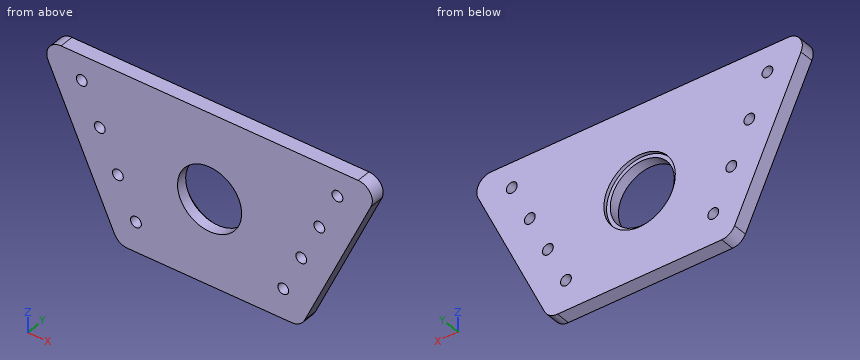
```python
from build123d import *

# Parameters (mm, degrees)
SKETCH1_R           = 14.2875
BOSS_EXTRUDE1_DEPTH = 6.35
SKETCH2_R           = 2.413
CUT_EXTRUDE1_DEPTH  = 86.430512699
FILLET1_R           = 6.35
SKETCH3_R           = 15.9385
CUT_EXTRUDE2_DEPTH  = 1.5875


with BuildPart() as part:
    # Sketch1 → Boss-Extrude1 (new body)
    with BuildSketch(Plane(origin=(0, 0, 0), x_dir=(1, 0, 0), z_dir=(0, 1, 0))):
        Polygon((-40.667356449, 38.1), (40.667356449, 38.1), (76.2, -38.1), (-76.2, -38.1), align=None)
        with Locations(Location((0, 0, 0), (0, 0, 270))):
            Circle(SKETCH1_R, mode=Mode.SUBTRACT)
    extrude(amount=BOSS_EXTRUDE1_DEPTH)

    # Sketch2 → Cut-Extrude1 (cut, through all)
    with BuildSketch(Plane(origin=(0, 6.35, 0), x_dir=(1, 0, 0), z_dir=(0, 1, 0))):
        with Locations(Location((-57.005256578, -26.9875, 0), (0, 0, 270))):
            Circle(SKETCH2_R)
        with Locations(Location((-48.954378692, -9.722336657, 0), (0, 0, 270))):
            Circle(SKETCH2_R)
        with Locations(Location((-40.903500806, 7.542826686, 0), (0, 0, 270))):
            Circle(SKETCH2_R)
        with Locations(Location((-32.852622919, 24.807990029, 0), (0, 0, 270))):
            Circle(SKETCH2_R)
        with Locations(Location((32.852622919, 24.807990029, 0), (0, 0, 90))):
            Circle(SKETCH2_R)
        with Locations(Location((40.903500806, 7.542826686, 0), (0, 0, 90))):
            Circle(SKETCH2_R)
        with Locations(Location((48.954378692, -9.722336657, 0), (0, 0, 90))):
            Circle(SKETCH2_R)
        with Locations(Location((57.005256578, -26.9875, 0), (0, 0, 90))):
            Circle(SKETCH2_R)
    extrude(amount=-CUT_EXTRUDE1_DEPTH, mode=Mode.SUBTRACT)

    # Fillet1
    fillet1_edges = [part.edges().sort_by_distance(p)[0] for p in [
        (-40.667356449, 3.175, -38.1),
        (40.667356449, 3.175, -38.1),
        (76.2, 3.175, 38.1),
        (-76.2, 3.175, 38.1),
    ]]
    fillet(fillet1_edges, radius=FILLET1_R)

    # Sketch3 → Cut-Extrude2 (cut)
    with BuildSketch(Plane(origin=(0, 6.35, 0), x_dir=(1, 0, 0), z_dir=(0, 1, 0))):
        with Locations(Location((0, 0, 0), (0, 0, 270))):
            Circle(SKETCH3_R)
    extrude(amount=-CUT_EXTRUDE2_DEPTH, mode=Mode.SUBTRACT)


solid = part.part
```
Input: part model. Units: mm. Frame: model coordinates. Give positions to 0.01 mm unless a question says otherwise; leave off trailing zeros. Order: outer loops, then holes, each group sorted by start corner. A loop starts at its lowest first (then second) coordinate and runs counter-clockwise, first axis right, second up. Notation, with made-up numbers: (10.25, -38) - (47.25, -38) arc R31 ccw to (47.25, -11) - close; hole circle Ø6 at (87.5, -7). An arc over 180 degrees is marked (long way). Use a Markdown table: item, result.
(1) Section query A-A (x = 0). Output: boundary loops of the cut face in (y, z).
Computed values:
| item | result |
|---|---|
| outline | (0, -38.1) - (6.35, -38.1) - (6.35, -15.94) - (4.76, -15.94) - (4.76, -14.29) - (0, -14.29) - close; (0, 14.29) - (4.76, 14.29) - (4.76, 15.94) - (6.35, 15.94) - (6.35, 38.1) - (0, 38.1) - close |
(2) Section query C-C (y = 2.25). State how many separate pieces and enclosed holes the cut face has, then the cut area to 3 significant figures.
Computed values:
| item | result |
|---|---|
| separate pieces | 1 |
| enclosed holes | 9 |
| area | 8,070 mm2 |
(3) Pin query (flat end, axial travel): pin 1 (23 mm diameter, centred on x = 0, z = 0, fed in from +Y); pin 2 (2 mm diameter, centred on y = 2, z = 27.5, fed in from -X). Return the tip coordinate at first contact, or that it passes through.
Computed values:
| item | result |
|---|---|
| pin 1 | passes through |
| pin 2 | stops at x = -71.72 |
(4) Line query: line 1 (X direction, y = 3, z = -9); line 2 (X direction, y = 0.75, z = -27); line 3 (X direction, y = 2.5, z = 25). Output: solid intervals per line, ascending. Write a range as from..to.
Computed values:
| item | result |
|---|---|
| line 1 | x = -54.24..-42.83, -38.98..-11.1, 11.1..38.98, 42.83..54.24 |
| line 2 | x = -45.84..-33.86, -31.84..31.84, 33.86..45.84 |
| line 3 | x = -70.09..-58.37, -55.64..55.64, 58.37..70.09 |
(5) Section query B-B (z = 0). Output: boundary loops of the cut face in (x, y), then the cut area to 3 significant figures.
Computed values:
| item | result |
|---|---|
| outline | (-58.43, 0) - (-14.29, 0) - (-14.29, 4.76) - (-15.94, 4.76) - (-15.94, 6.35) - (-58.43, 6.35) - close; (14.29, 0) - (58.43, 0) - (58.43, 6.35) - (15.94, 6.35) - (15.94, 4.76) - (14.29, 4.76) - close |
| area | 555 mm2 |
